```python
from build123d import *

# Parameters (mm, degrees)
F1_DEPTH = 50.8
F2_R     = 19.05
F3_DEPTH = 12.7
F4_DEPTH = 12.7


with BuildPart() as f1:
    # F0 (on Front) → F1 (new body)
    with BuildSketch(Plane.XZ):
        Polygon((-44.45, 5.3018676117), (-44.45, -25.4), (44.45, -25.4), (44.45, 0), (32.0377089083, 25.4), (-33.9801497757, 25.4), align=None)
        Polygon((-82.4199393392, -25.4), (-44.45, -25.4), (-44.45, 5.3018676117), (-83.6249068379, -4.5788856223), align=None)
    extrude(amount=F1_DEPTH)

    # F2 (on Front) → F3 (cut)
    with BuildSketch(Plane.XZ):
        with Locations((-42.0304983854, -18.3155424893)):
            Circle(F2_R)
        with BuildLine():
            ThreePointArc((5.4338427752, -18.3155424893), (24.4838427752, -37.3655424893), (43.5338427752, -18.3155424893))
            ThreePointArc((43.5338427752, -18.3155424893), (24.4838427752, 0.7344575107), (5.4338427752, -18.3155424893))
        make_face()
    extrude(amount=F3_DEPTH, mode=Mode.SUBTRACT)



with BuildPart() as f4:
    # F2 (on Front) → F4 (new body)
    with BuildSketch(Plane.XZ):
        with BuildLine():
            ThreePointArc((5.4338427752, -18.3155424893), (24.4838427752, -37.3655424893), (43.5338427752, -18.3155424893))
            ThreePointArc((43.5338427752, -18.3155424893), (24.4838427752, 0.7344575107), (5.4338427752, -18.3155424893))
        make_face()
    extrude(amount=F4_DEPTH)


with BuildPart() as f4b:
    # F2 (on Front) → F4, piece 2 (new body)
    with BuildSketch(Plane.XZ):
        with Locations((-42.0304983854, -18.3155424893)):
            Circle(F2_R)
    extrude(amount=F4_DEPTH)


with BuildPart() as f1_1:
    add(f1.part)

    add(f4.part)  # F5 merges F4

    add(f4b.part)  # F5 merges F4b
    # F5: F4b, F4 across plane
    add(f4b.part.mirror(Plane.XZ))
    add(f4.part.mirror(Plane.XZ))


solid = f1_1.part
```
For this review, take the finished solid that the model builds, in its own axes (mm). A direction names the side the tool comes from. Coordinates: 2 decimals unless noted, no trailing zeros. Write each loop counter-clockwise with the first axis right and the second up, starting at its lowest first coordinate (ties: lowest second). Pieces come first, ordered by that corner, then holes.
(1) Add section B-B on y = -38.5. Give the boundary of the cut face in (x, z), then the cut area to 3 significant figures.
(2) For pin 1 Ø3.5 at (x, z) = (-39.5, -29) entering from -Y; pin 2 Ø1.5 at (y, z) = (-39.5, 13.5) entering from +X; pin 3 Ø4 at (y, z) = (-0.5, -27.5) entering from +X, all flat-tipped, find the tip position at first contact; note any pin that passes through.
(3) Tool access review of faces 4 (the face through (-42, -12.7, -30)), 5 (the face through (-46.16, 2.644, -36.913)), 6 (the face through (-39.142, -25.044, 15.492)): name each direction out of +Z, -Z, +X, -X, +Y, -Y from which nothing blocks a thin tool from reaching the whole face with its end or side.
(4) Add section C-C on x = -27.5. Give the boundary of the cut face in (y, z).
(5) Wall thickness on probe 1 along Y at (x, z) = (-6, -2); probe 2 along Z at (x, y) = (25.5, -34); probe 3 along X at (y, z) = (9, -17): over which ranges is each line inside the solid? List them lowest first.
(6) Add section D-D on z = -9. Give the boundary of the cut face in (x, y).
(7) The part is to be moulded in two halves that separate along X. For faces 1 (the face through (-63.76, -25.04, 0.43)), 2 (the face through (33.27, 2.64, -35.22)), 3 (the face through (-42, 12.7, -18)), say which applies: +X half, -X half, draft (parallel to the pull), parting line (faces both ways), or undercut.
(8) Add section A-A on z = -28. Give the boundary of the cut face in (x, y), then the cut area to 3 significant figures.
Answer sheet:
1. outline: (-83.62, -4.58) - (-82.42, -25.4) - (44.45, -25.4) - (44.45, 0) - (32.04, 25.4) - (-33.98, 25.4) - (-44.45, 5.3) - close
1. area: 5,250 mm2
2. pin 1: stops at y = -12.7
2. pin 2: stops at x = 38.22
2. pin 3: stops at x = 42.13
3. face 4: -Z, +X, -X, -Y
3. face 5: +Y
3. face 6: +Z, -X, +Y, -Y
4. outline: (-50.8, -25.4) - (-12.7, -25.4) - (-12.7, -30.63) - (12.7, -30.63) - (12.7, -6) - (0, -6) - (0, 25.4) - (-50.8, 25.4) - close
5. probe 1: y = -50.8 to 0
5. probe 2: z = -25.4 to 25.4
5. probe 3: x = -61.04 to -23.03, 5.48 to 43.49
6. outline: (-83.37, -50.8) - (44.45, -50.8) - (44.45, 0) - (41.1, 0) - (41.1, 12.7) - (7.87, 12.7) - (7.87, 0) - (-25.41, 0) - (-25.41, 12.7) - (-58.65, 12.7) - (-58.65, 0) - (-83.37, 0) - close
7. face 1: -X half
7. face 2: undercut
7. face 3: draft
8. outline: (-58.44, -12.7) - (-25.63, -12.7) - (-25.63, 12.7) - (-58.44, 12.7) - close; (8.08, -12.7) - (40.89, -12.7) - (40.89, 12.7) - (8.08, 12.7) - close
8. area: 1,670 mm2
